from build123d import *

# Parameters (mm, degrees)
BOSS_EXTRU_2_DEPTH      = 9
ESQUISSE3_W             = 51.8612703
ESQUISSE3_H             = 63
BOSS_EXTRU_3_DEPTH      = 3
ESQUISSE4_W             = 10
ESQUISSE4_H             = 3.4
ENL_V_MAT_EXTRU_1_DEPTH = 7
ESQUISSE5_W             = 3.2
ESQUISSE5_H             = 3
BOSS_EXTRU_4_DEPTH      = 63
CHANFREIN1_SIZE         = 1
CHANFREIN2_SIZE         = 2
CONG_1_R                = 1
CONG_2_R                = 1
CHANFREIN4_SIZE         = 1
CONG_4_R                = 1
CONG_5_R                = 1
ESQUISSE6_W             = 6.7
ESQUISSE6_H             = 1
BOSS_EXTRU_5_DEPTH      = 10
ESQUISSE7_W             = 25.281431527
ESQUISSE7_H             = 35.175981147
ENL_V_MAT_EXTRU_2_DEPTH = 79


with BuildPart() as part:
    # Esquisse2 → Boss.-Extru.2 (new body)
    with BuildSketch(Plane.XY):
        Polygon((-9.3, -31.5), (-9.3, -21.5), (-21.5, -21.5), (-21.5, 21.5), (21.5, 21.5), (21.5, -21.5), (9.3, -21.5), (9.3, -31.5), (25.93063515, -31.5), (25.93063515, 31.5), (-25.93063515, 31.5), (-25.93063515, -31.5), align=None)
    extrude(amount=BOSS_EXTRU_2_DEPTH)

    # Esquisse3 → Boss.-Extru.3 (add)
    with BuildSketch(Plane(origin=(0, 0, 0), x_dir=(-1, 0, 0), z_dir=(0, 0, -1))):
        Rectangle(ESQUISSE3_W, ESQUISSE3_H)
    extrude(amount=BOSS_EXTRU_3_DEPTH)

    # Esquisse4 → Enlèv. mat.-Extru.1 (cut)
    with BuildSketch(Plane.XY.offset(9)):
        with Locations((-16.5, -26.695538472)):
            Rectangle(ESQUISSE4_W, ESQUISSE4_H)
        with Locations((16.5, -26.695538472)):
            Rectangle(ESQUISSE4_W, ESQUISSE4_H)
        with Locations((16.5, 26.695538472)):
            Rectangle(ESQUISSE4_W, ESQUISSE4_H)
        with Locations((-16.5, 26.695538472)):
            Rectangle(ESQUISSE4_W, ESQUISSE4_H)
    extrude(amount=-ENL_V_MAT_EXTRU_1_DEPTH, mode=Mode.SUBTRACT)

    # Esquisse5 → Boss.-Extru.4 (add)
    with BuildSketch(Plane(origin=(0, 31.5, 0), x_dir=(1, 0, 0), z_dir=(0, 1, 0))):
        Polygon((-29.13063515, 0), (-29.13063515, 3), (-31.63063515, 3), (-31.63063515, -6), (-29.13063515, -6), align=None)
        with Locations((-27.53063515, 1.5)):
            Rectangle(ESQUISSE5_W, ESQUISSE5_H)
        with Locations((27.53063515, 1.5)):
            Rectangle(ESQUISSE5_W, ESQUISSE5_H)
        Polygon((29.13063515, 3), (29.13063515, 0), (29.13063515, -6), (31.63063515, -6), (31.63063515, 3), align=None)
    extrude(amount=-BOSS_EXTRU_4_DEPTH)

    # Chanfrein1
    chanfrein1_edges = [part.edges().sort_by_distance(p)[0] for p in [
        (21.5, -21.5, 4.5),
        (21.5, 21.5, 4.5),
        (-21.5, 21.5, 4.5),
        (-21.5, -21.5, 4.5),
    ]]
    chamfer(chanfrein1_edges, length=CHANFREIN1_SIZE)

    # Chanfrein2
    chanfrein2_edges = [part.edges().sort_by_distance(p)[0] for p in [
        (-31.63063515, 0, -3),
        (31.63063515, 0, -3),
        (0, -31.5, -3),
        (0, 31.5, -3),
    ]]
    chamfer(chanfrein2_edges, length=CHANFREIN2_SIZE)

    # Congé1
    cong_1_edges = [part.edges().sort_by_distance(p)[0] for p in [
        (-25.93063515, 0, 0),
        (-29.13063515, 0, 0),
        (-29.13063515, 0, 6),
        (-31.63063515, 0, 6),
        (25.93063515, 0, 0),
        (29.13063515, 0, 0),
        (29.13063515, 0, 6),
        (31.63063515, 0, 6),
    ]]
    fillet(cong_1_edges, radius=CONG_1_R)

    # Congé2
    cong_2_edges = [part.edges().sort_by_distance(p)[0] for p in [
        (-31.63063515, 31.5, 2),
        (31.63063515, 31.5, 2),
        (30.38063515, -31.5, 6),
        (30.38063515, 31.5, 6),
        (-30.38063515, 31.5, 6),
        (-29.13063515, 31.5, 3),
        (-27.53063515, 31.5, 0),
        (27.53063515, 31.5, 0),
        (29.13063515, 31.5, 3),
        (-31.337741931, 31.5, 5.707106781),
        (-29.423528369, 31.5, 5.707106781),
        (29.423528369, 31.5, 5.707106781),
        (31.337741931, 31.5, 5.707106781),
        (31.63063515, -31.5, 2),
        (-31.63063515, -31.5, 2),
        (29.13063515, -31.5, 3),
        (27.53063515, -31.5, 0),
        (-27.53063515, -31.5, 0),
        (-29.13063515, -31.5, 3),
        (-30.38063515, -31.5, 6),
        (-31.337741931, -31.5, 5.707106781),
        (-29.423528369, -31.5, 5.707106781),
        (29.423528369, -31.5, 5.707106781),
        (31.337741931, -31.5, 5.707106781),
        (28.837741931, 31.5, 0.292893219),
        (28.837741931, -31.5, 0.292893219),
        (26.223528369, 31.5, 0.292893219),
        (26.223528369, -31.5, 0.292893219),
        (-28.837741931, 31.5, 0.292893219),
        (-28.837741931, -31.5, 0.292893219),
        (-26.223528369, 31.5, 0.292893219),
        (-26.223528369, -31.5, 0.292893219),
        (-25.93063515, -31.5, 5),
        (-25.93063515, 31.5, 5),
        (25.93063515, 31.5, 5),
        (25.93063515, -31.5, 5),
    ]]
    fillet(cong_2_edges, radius=CONG_2_R - 0.0001)  # a hair under: the kernel refuses the full size

    # Chanfrein4
    chanfrein4_edges = [part.edges().sort_by_distance(p)[0] for p in [
        (-9.3, -31.5, 4.5),
        (9.3, -31.5, 4.5),
        (9.3, -21.5, 4.5),
        (-9.3, -21.5, 4.5),
    ]]
    chamfer(chanfrein4_edges, length=CHANFREIN4_SIZE)

    # Congé4
    cong_4_edges = [part.edges().sort_by_distance(p)[0] for p in [
        (-21.5, 0, 9),
        (-15.4, -21.5, 9),
        (21.5, 0, 9),
        (0, 21.5, 9),
        (-21, -21, 9),
        (21, -21, 9),
        (21, 21, 9),
        (-21, 21, 9),
        (0, 31.5, 9),
        (-17.615367575, -31.5, 9),
        (-25.93063515, 0, 9),
        (25.93063515, 0, 9),
        (25.63777122, 31.207136071, 9),
        (25.63777122, -31.207136071, 9),
        (-25.63777122, -31.207136071, 9),
        (-25.63777122, 31.207136071, 9),
        (17.615367575, -31.5, 9),
        (9.3, -26.5, 9),
        (-9.3, -26.5, 9),
        (15.4, -21.5, 9),
        (-9.8, -22, 9),
        (9.8, -22, 9),
        (-9.8, -31, 9),
        (9.8, -31, 9),
        (-16.5, 28.395538472, 9),
        (-11.5, 26.695538472, 9),
        (-21.5, 26.695538472, 9),
        (-16.5, 24.995538472, 9),
        (21.5, 26.695538472, 9),
        (16.5, 24.995538472, 9),
        (16.5, 28.395538472, 9),
        (11.5, 26.695538472, 9),
        (16.5, -28.395538472, 9),
        (11.5, -26.695538472, 9),
        (21.5, -26.695538472, 9),
        (16.5, -24.995538472, 9),
        (-21.5, -26.695538472, 9),
        (-16.5, -24.995538472, 9),
        (-16.5, -28.395538472, 9),
        (-11.5, -26.695538472, 9),
    ]]
    fillet(cong_4_edges, radius=CONG_4_R - 0.0001)  # a hair under: the kernel refuses the full size

    # Congé5
    cong_5_edges = [part.edges().sort_by_distance(p)[0] for p in [
        (9.3, -26.5, 0),
        (-9.3, -26.5, 0),
        (9.8, -31, 0),
        (-9.8, -31, 0),
    ]]
    fillet(cong_5_edges, radius=CONG_5_R)

    # Esquisse6 → Boss.-Extru.5 (add)
    with BuildSketch(Plane.XZ.offset(31.5)):
        with BuildLine():
            Line((-24.93063515, 1), (-24.93063515, 5))
            Line((-24.93063515, 5), (-31.63063515, 5))
            Line((-31.63063515, 5), (-31.63063515, -1))
            Line((-31.63063515, -1), (-26.93063515, -1))
            ThreePointArc((-26.93063515, -1), (-25.516421587, -0.414213562), (-24.93063515, 1))
        make_face()
        with Locations((-28.28063515, 5.5)):
            Rectangle(ESQUISSE6_W, ESQUISSE6_H)
        with BuildLine():
            Line((31.63063515, -1), (31.63063515, 5))
            Line((31.63063515, 5), (24.93063515, 5))
            Line((24.93063515, 5), (24.93063515, 1))
            ThreePointArc((24.93063515, 1), (25.516421587, -0.414213562), (26.93063515, -1))
            Line((26.93063515, -1), (31.63063515, -1))
        make_face()
        with Locations((28.28063515, 5.5)):
            Rectangle(ESQUISSE6_W, ESQUISSE6_H)
    extrude(amount=-BOSS_EXTRU_5_DEPTH)

    # Esquisse7 → Enlèv. mat.-Extru.2 (cut)
    with BuildSketch(Plane(origin=(31.63063515, 0, 0), x_dir=(0, 0, -1), z_dir=(1, 0, 0))):
        with Locations((3.640715764, 17.587990574)):
            Rectangle(ESQUISSE7_W, ESQUISSE7_H)
    extrude(amount=-ENL_V_MAT_EXTRU_2_DEPTH, mode=Mode.SUBTRACT)


solid = part.part
The model under review builds one solid part; all positions refer to its coordinate system, in mm. A direction names the side the tool comes from. Round coordinates to 2 decimals unless told otherwise and drop trailing zeros. Order: outer loops, then holes, each group sorted by start corner. A loop starts at its lowest first (then second) coordinate and runs counter-clockwise, first axis right, second up. Notation, with made-up numbers: (73.25, -38) -> (105.25, -38) arc R26 ccw to (105.25, -17) -> close; hole circle Ø2 at (12, 78.25). An arc over 180 degrees is marked (long way). Use CSV: the item, a comma, the result in double quotes. Start each with the question number.
(1) Tool access review of faces 4 (the face through (-17, -28.396, 5)), 5 (the face through (-15, -21.5, 4)), 6 (the face through (-9.916, -30.87, 8.565)): name each direction out of +Z, -Z, +X, -X, +Y, -Y from which nothing blocks a thin tool from reaching the whole face with its end or side.
(2) Wall thickness on probe 1 along X at (y, z) = (-6, 4.5); probe 2 along X at (y, z) = (-28, 6.5); probe 3 along X at (y, z) = (-14, 7): over which ranges is each line inside the solid? List them lowest first. Write a range as from..to.
(3) Consider section B-B on x = 16. Write out the cut boundary in (y, z), and give its area (3 significant figures).
(4) Insertion check: pin 1 (1.5 mm diameter, centred on x = 17.5, y = -20, fed in from +Z); pin 2 (5 mm diameter, centred on x = 15.5, z = 6, fed in from +Y); pin 3 (1 mm diameter, centred on x = 17, y = -26, fed in from +Z). Each pin has a flat end and moves straight along its axis. Give the tip position at first contact, or say it passes through.
(5) Consider section A-A on z = 7. Write out the cut boundary in (x, y).
(6) Mouldability with a two-part tool opening along Y and no side actions: class faces 1 (the face through (-27.5, -10.6, 0)), 2 (the face through (-17, -27, 2)), 3 (the face through (-9.93, -22.116, 8.565)) as pulls with the +Y half, pulls with the -Y half, needs draft (parallel to the pull), parting line crosses it, or undercut.
Responses:
1,face 4,"+Z"
1,face 5,"+Z, +Y"
1,face 6,"+Z, -Y"
2,probe 1,"-31.63..-29.13, -25.93..-21.5, 21.5..25.93, 29.13..31.63"
2,probe 2,"-25.93..-21.5, -11.5..-9.3, 9.3..11.5, 21.5..25.93"
2,probe 3,"-25.93..-21.5, 21.5..25.93"
3,outline,"(-31.5, -1) -> (-29.5, -3) -> (0, -3) -> (0, 0) -> (-21.5, 0) -> (-21.5, 8) arc R1 ccw to (-22.5, 9) -> (-24, 9) arc R1 ccw to (-25, 8) -> (-25, 2) -> (-28.4, 2) -> (-28.4, 8) arc R1 ccw to (-29.4, 9) -> (-30.5, 9) arc R1 ccw to (-31.5, 8) -> close"
3,area,"158 mm²"
4,pin 1,"z = 0"
4,pin 2,"y = -21.5"
4,pin 3,"z = 2"
5,outline,"(-25.93, -30.5) arc R1 ccw to (-24.93, -31.5) -> (-10.3, -31.5) -> (-9.3, -30.5) -> (-9.3, -22.5) -> (-10.3, -21.5) -> (-20.5, -21.5) -> (-21.5, -20.5) -> (-21.5, 0) -> (-25.93, 0) -> close; (9.3, -30.5) -> (10.3, -31.5) -> (24.93, -31.5) arc R1 ccw to (25.93, -30.5) -> (25.93, 0) -> (21.5, 0) -> (21.5, -20.5) -> (20.5, -21.5) -> (10.3, -21.5) -> (9.3, -22.5) -> close; hole (-21.5, -28.4) -> (-11.5, -28.4) -> (-11.5, -25) -> (-21.5, -25) -> close; hole (11.5, -28.4) -> (21.5, -28.4) -> (21.5, -25) -> (11.5, -25) -> close"
6,face 1,"needs draft"
6,face 2,"undercut"
6,face 3,"pulls with the +Y half"
